Design review of the part built by this model. Coordinates are the model's own, in mm. A direction names the side the tool comes from. Give positions to 0.01 mm unless a question says otherwise; leave off trailing zeros. Loops run counter-clockwise (first coordinate to the right, second up) from the corner with the lowest first, then second, coordinate; pieces in that order, holes last.
from build123d import *

# Parameters (mm, degrees)
F1_DEPTH = 300
F2_R     = 75
F3_DEPTH = 50
F4_W     = 218
F4_H     = 371.600151062
F5_DEPTH = 10
F7_DEPTH = 218
F8_R     = 75
F9_DEPTH = 50


with BuildPart() as f1:
    # F0 (on Right) → F1 (new body)
    with BuildSketch(Plane.YZ):
        Polygon((350, 75), (350, 150), (-350, 150), (-350, -150), (350, -150), (350, 0), align=None)
    extrude(amount=F1_DEPTH)

    # F2 (on face) → F3 (join)
    with BuildSketch(Plane(origin=(0, 350, 0), x_dir=(-1, 0, 0), z_dir=(0, 1, 0))):
        with Locations((-150, 0)):
            Circle(F2_R)
    extrude(amount=F3_DEPTH)

    # F4 (on face) → F5 (join)
    with BuildSketch(Plane(origin=(0, 0, -150), x_dir=(1, 0, 0), z_dir=(0, 0, -1))):
        with Locations((150, 0)):
            Rectangle(F4_W, F4_H)
    extrude(amount=F5_DEPTH)

    # F6 (on face) → F7 (join)
    with BuildSketch(Plane(origin=(41, 0, 0), x_dir=(0, -1, 0), z_dir=(-1, 0, 0))):
        Polygon((185.800075531, -160), (-185.800075531, -160), (-106, -417.9378761354), (106, -417.9378761354), align=None)
    extrude(amount=-F7_DEPTH)

    # F8 (on face) → F9 (join)
    with BuildSketch(Plane.XZ.offset(350)):
        with Locations((150, 0)):
            Circle(F8_R)
    extrude(amount=F9_DEPTH)


solid = f1.part
Q1. Take a section at D-D (x = 113). Give the boundary of the cut face in (y, z), plus the area to 3 significant figures.
Results:
outline: (-400, -65.24) - (-350, -65.24) - (-350, -150) - (-185.8, -150) - (-185.8, -160) - (-106, -417.94) - (106, -417.94) - (185.8, -160) - (185.8, -150) - (350, -150) - (350, -65.24) - (400, -65.24) - (400, 65.24) - (350, 65.24) - (350, 150) - (-350, 150) - (-350, 65.24) - (-400, 65.24) - close
area: 302,000 mm2
Q2. Take a section at A-A (z = 0). Give the boundary of the cut face in (x, y), plus the area to 3 significant figures.
Results:
outline: (0, -350) - (75, -350) - (75, -400) - (225, -400) - (225, -350) - (300, -350) - (300, 350) - (225, 350) - (225, 400) - (75, 400) - (75, 350) - (0, 350) - close
area: 225,000 mm2
Q3. Tool access review of faces 1 (the face through (81, -350, 35)), 2 (the face through (81, 350, -35)), 3 (the face through (259, 3, -282)), 4 (the face through (41, 3, -282)), 5 (the face through (148, 5, 150)): name each direction out of +Z, -Z, +X, -X, +Y, -Y from which nothing blocks a thin tool from reaching the whole face with its end or side.
Results:
face 1: -Y
face 2: +Y
face 3: -Z, +X, +Y, -Y
face 4: -Z, -X, +Y, -Y
face 5: +Z, +X, -X, +Y, -Y
Q4. Take a section at B-B (y = -53). Give the boundary of the cut face in (x, z), plus the area to 3 significant figures.
Results:
outline: (0, -150) - (41, -150) - (41, -417.94) - (259, -417.94) - (259, -150) - (300, -150) - (300, 150) - (0, 150) - close
area: 148,000 mm2
Q5. Insertion check: pin 1 (11 mm diameter, centred on x = 178, z = -154.5, fed in from +Y); pin 2 (11 mm diameter, centred on x = 161, z = -154.5, fed in from -Y); pin 3 (10 mm diameter, centred on x = 156, y = 225.5, fed in from -Z). Each pin has a flat end and moves straight along its axis. Give the tip position at first contact, or say it passes through.
Results:
pin 1: stops at y = 350
pin 2: stops at y = -350
pin 3: stops at z = -150
Q6. Wall thickness on line 1 (X direction, y = 20, z = -197.5); line 2 (Z direction, x = 286, y = 237.5); line 3 (Y direction, x = 273, z = -115): over which ranges is each line inside the solid? List them lowest first.
Results:
line 1: x = 41 to 259
line 2: z = -150 to 150
line 3: y = -350 to 350
Q7. Take a section at C-C (x = 150). Give the boundary of the cut face in (y, z).
Results:
outline: (-400, -75) - (-350, -75) - (-350, -150) - (-185.8, -150) - (-185.8, -160) - (-106, -417.94) - (106, -417.94) - (185.8, -160) - (185.8, -150) - (350, -150) - (350, -75) - (400, -75) - (400, 75) - (350, 75) - (350, 150) - (-350, 150) - (-350, 75) - (-400, 75) - close
